Print and shaded views of the part. All mm, measured from the part's lowest x, y and z. A direction names the side the tool comes from. Round coordinates to 2 decimals unless told otherwise and drop trailing zeros. Write each loop counter-clockwise with the first axis right and the second up, starting at its lowest first coordinate (ties: lowest second). Pieces come first, ordered by that corner, then holes.
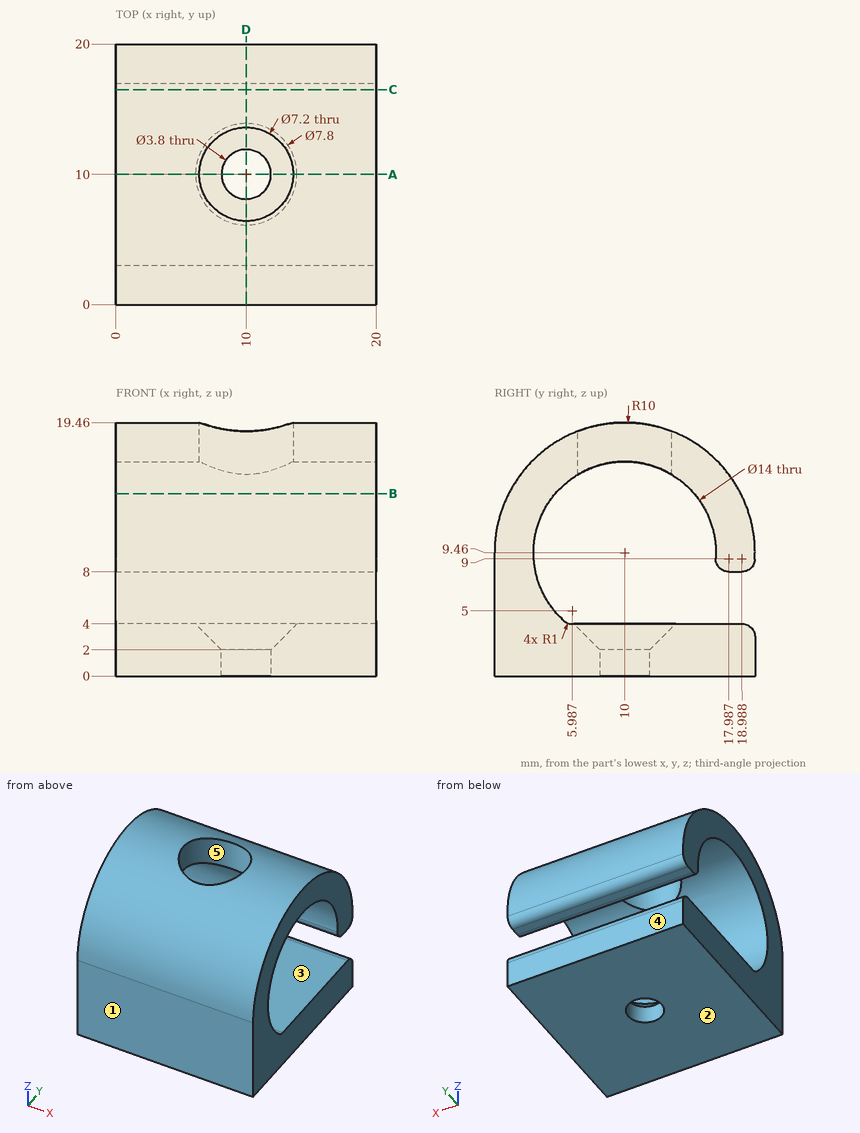
1) Slice it at A-A (y = 10). Write the cut outline in (x, z).
Results:
outline: (0, 0) - (8.1, 0) - (8.1, 2) - (6.1, 4) - (0, 4) - close; (0, 16.46) - (6.4, 16.46) - (6.4, 19.46) - (0, 19.46) - close; (11.9, 0) - (20, 0) - (20, 4) - (13.9, 4) - (11.9, 2) - close; (13.6, 16.46) - (20, 16.46) - (20, 19.46) - (13.6, 19.46) - close
2) Wall check: L1, parallel to Z at x = 6, y = 10; L2, parallel to Y at x = 10, z = 1.1; L3, parallel to Y at x = 3.25, z = 9.5. Give the ranges that are in metal, low to high.
Results:
L1: z = 0 to 4, 16.46 to 19.46
L2: y = 0 to 8.1, 11.9 to 20
L3: y = 0 to 3, 17 to 20
3) Slice it at D-D (x = 10). Write the cut outline in (y, z).
Results:
outline: (0, 0) - (8.1, 0) - (8.1, 2) - (6.1, 4) - (5.99, 4) arc R1 cw to (5.32, 4.26) arc R7 cw to (6.4, 15.46) - (6.4, 18.79) arc R10 ccw to (0, 9.46) - close; (11.9, 0) - (20, 0) - (20, 3) arc R1 ccw to (19, 4) - (13.9, 4) - (11.9, 2) - close; (13.6, 15.46) arc R7 cw to (16.99, 9.06) arc R1 ccw to (17.99, 8) - (18.99, 8) arc R1 ccw to (19.99, 8.95) arc R10 ccw to (13.6, 18.79) - close
4) Slice it at C-C (y = 16.5). Write the cut outline in (x, z), plus the area to 3 significant figures.
Results:
outline: (0, 0) - (20, 0) - (20, 4) - (0, 4) - close; (0, 12.06) - (20, 12.06) - (20, 17.06) - (0, 17.06) - close
area: 180 mm2
5) Pin check, flat tips, straight feed: pin 1 Ø4 at (x, y) = (8, 16) entering from +Z (1 decimal); pin 2 Ø3 at (x, z) = (7, 13.5) entering from +Y; pin 3 Ø6.5 at (x, y) = (6.5, 15.5) entering from +Z. Stop position of each tip, or through.
Results:
pin 1: stops at z = 18.6
pin 2: stops at y = 19.67
pin 3: stops at z = 19.2
6) Which spindle directions (+Z, -Z, +X, -X, +Y, -Y) get a long thin tool onto all of the face, cutting with end or side? Do the marked faces 4 and 5. Say none if no direction does.
Results:
face 4: +Z, -Z, +X, -X, +Y
face 5: +Z
7) Slice it at B-B (z = 14). Write the cut outline in (x, y), plus the area to 3 significant figures.
Results:
outline: (0, 1.09) - (20, 1.09) - (20, 4.67) - (0, 4.67) - close; (0, 15.33) - (20, 15.33) - (20, 18.91) - (0, 18.91) - close
area: 143 mm2
8) Mould opens along Z. For the marked faces 1, 2 and 3 say: released by +Z, released by -Z, zero draft, split by the parting line, or undercut.
Results:
face 1: zero draft
face 2: released by -Z
face 3: undercut
